```python
from build123d import *

# Parameters (mm, degrees)
ESQUISSE1_W             = 40
ESQUISSE1_H             = 20
BOSS_EXTRU_1_DEPTH      = 2
ESQUISSE2_W             = 40
ESQUISSE2_H             = 2
BOSS_EXTRU_2_DEPTH      = 18
ESQUISSE3_R             = 3
ENL_V_MAT_EXTRU_1_DEPTH = 18
ESQUISSE4_R             = 3
ENL_V_MAT_EXTRU_2_DEPTH = 18
ESQUISSE5_R             = 3
ENL_V_MAT_EXTRU_3_DEPTH = 18
ESQUISSE6_R             = 3
ENL_V_MAT_EXTRU_4_DEPTH = 18
ESQUISSE7_W             = 6
ESQUISSE7_H             = 18
BOSS_EXTRU_3_DEPTH      = 18
ESQUISSE8_R             = 3
ENL_V_MAT_EXTRU_5_DEPTH = 18
CHANFREIN1_SIZE         = 3
CONG_1_R                = 3


with BuildPart() as part:
    # Esquisse1 → Boss.-Extru.1 (new body)
    with BuildSketch(Plane.XY):
        with Locations((-20, 10)):
            Rectangle(ESQUISSE1_W, ESQUISSE1_H)
    extrude(amount=BOSS_EXTRU_1_DEPTH)

    # Esquisse2 → Boss.-Extru.2 (add)
    with BuildSketch(Plane.XY.offset(2)):
        with Locations((-20, 1)):
            Rectangle(ESQUISSE2_W, ESQUISSE2_H)
    extrude(amount=BOSS_EXTRU_2_DEPTH)

    # Esquisse3 → Enlèv. mat.-Extru.1 (cut)
    with BuildSketch(Plane.XY.offset(2)):
        with Locations((-6, 10)):
            Circle(ESQUISSE3_R)
    extrude(amount=-ENL_V_MAT_EXTRU_1_DEPTH, mode=Mode.SUBTRACT)

    # Esquisse4 → Enlèv. mat.-Extru.2 (cut)
    with BuildSketch(Plane.XY.offset(2)):
        with Locations((-25, 10)):
            Circle(ESQUISSE4_R)
    extrude(amount=-ENL_V_MAT_EXTRU_2_DEPTH, mode=Mode.SUBTRACT)

    # Esquisse5 → Enlèv. mat.-Extru.3 (cut)
    with BuildSketch(Plane(origin=(0, 2, 0), x_dir=(1, 0, 0), z_dir=(0, 1, 0))):
        with Locations(Location((-6, -10, 0), (0, 0, 180))):  # turned: the seam where the file's is
            Circle(ESQUISSE5_R)
    extrude(amount=-ENL_V_MAT_EXTRU_3_DEPTH, mode=Mode.SUBTRACT)

    # Esquisse6 → Enlèv. mat.-Extru.4 (cut)
    with BuildSketch(Plane(origin=(0, 2, 0), x_dir=(1, 0, 0), z_dir=(0, 1, 0))):
        with Locations(Location((-25, -10, 0), (0, 0, 180))):  # turned: the seam where the file's is
            Circle(ESQUISSE6_R)
    extrude(amount=-ENL_V_MAT_EXTRU_4_DEPTH, mode=Mode.SUBTRACT)

    # Esquisse7 → Boss.-Extru.3 (add)
    with BuildSketch(Plane(origin=(0, 2, 0), x_dir=(1, 0, 0), z_dir=(0, 1, 0))):
        with Locations((-37, -11)):
            Rectangle(ESQUISSE7_W, ESQUISSE7_H)
    extrude(amount=BOSS_EXTRU_3_DEPTH)

    # Esquisse8 → Enlèv. mat.-Extru.5 (cut)
    with BuildSketch(Plane.ZY.offset(40)):
        with Locations((14, 14)):
            Circle(ESQUISSE8_R)
    extrude(amount=-ENL_V_MAT_EXTRU_5_DEPTH, mode=Mode.SUBTRACT)

    # Chanfrein1
    chanfrein1_edges = [part.edges().sort_by_distance(p)[0] for p in [
        (-37, 20, 20),
    ]]
    chamfer(chanfrein1_edges, length=CHANFREIN1_SIZE)

    # Congé1
    cong_1_edges = [part.edges().sort_by_distance(p)[0] for p in [
        (-34, 11, 2),
    ]]
    fillet(cong_1_edges, radius=CONG_1_R)


solid = part.part
```
Geometry: final body of the model. Coordinates: model frame, mm. A direction names the side the tool comes from. Coordinates: 2 decimals unless noted, no trailing zeros. Order: outer loops, then holes, each group sorted by start corner. A loop starts at its lowest first (then second) coordinate and runs counter-clockwise, first axis right, second up. Notation, with made-up numbers: (-23, -31.75) - (24, -31.75) arc R15 ccw to (24, -21.75) - close; hole circle Ø4 at (78, -15). An arc over 180 degrees is marked (long way). Return JSON: item names as keys, results as strings. Group by question number.
1. Pin query (flat end, axial travel): pin 1 (7 mm diameter, centred on x = -6, z = 10, fed in from +Y); pin 2 (9.5 mm diameter, centred on y = 14, z = 14, fed in from +X); pin 3 (5.5 mm diameter, centred on x = -12, y = 8, fed in from +Z). Return the tip coordinate at first contact, or that it passes through.
2. Cut plane A-A (y = 14). Output: boundary loops of the cut face in (x, z).
3. Pull-direction query (Y, two-part tool) for faces 1 (the face through (-20, 10, 0)), 2 (the face through (-3.14, 10.9, 1.01)), 3 (the face through (-37, 12.2, 11.6)), 4 (the face through (-30.5, 20, 1.5)); classes: pulls with the +Y half, pulls with the -Y half, needs draft (parallel to the pull), parting line crosses it, or undercut.
4. Cut plane D-D (x = -6). Output: boundary loops of the cut face in (y, z).
5. Material intervals for line 1 along Y through (x, z) = (-6, 0.9); line 2 along X through (y, z) = (9, 16), sorted ascending. Write a range as [from, to].
6. Set-up query: faces 5 (the face through (-22, 1, 10)), 6 (the face through (-34, 11, 13)). Return all of +Z, -Z, +X, -X, +Y, -Y with unobstructed straight access to the full face (end or side cutting, diameter ignored); none if empty.
7. Cut plane C-C (y = 10). Output: boundary loops of the cut face in (x, z).
8. Cut plane B-B (z = 14). Output: boundary loops of the cut face in (x, y), plus the area to 3 significant figures.
Resolved:
{
 "1": {"pin 1": "stops at y = 2", "pin 2": "stops at x = -34", "pin 3": "stops at z = 2"},
 "2": {"outline": "(-40, 0) - (0, 0) - (0, 2) - (-31, 2) arc R3 cw to (-34, 5) - (-34, 11) - (-40, 11) - close; (-40, 17) - (-34, 17) - (-34, 20) - (-40, 20) - close"},
 "3": {"face 1": "needs draft", "face 2": "undercut", "face 3": "undercut", "face 4": "pulls with the +Y half"},
 "4": {"outline": "(0, 0) - (7, 0) - (7, 2) - (2, 2) - (2, 7) - (0, 7) - close; (0, 13) - (2, 13) - (2, 20) - (0, 20) - close; (13, 0) - (20, 0) - (20, 2) - (13, 2) - close"},
 "5": {"line 1": "y = [0, 7], [13, 20]", "line 2": "x = [-40, -34]"},
 "6": {"face 5": "+Y, -Y", "face 6": "+Z, +X, +Y"},
 "7": {"outline": "(-40, 0) - (-28, 0) - (-28, 2) - (-31, 2) arc R3 cw to (-34, 5) - (-34, 20) - (-40, 20) - close; (-22, 0) - (-9, 0) - (-9, 2) - (-22, 2) - close; (-3, 0) - (0, 0) - (0, 2) - (-3, 2) - close"},
 "8": {"outline": "(-40, 0) - (0, 0) - (0, 2) - (-34, 2) - (-34, 11) - (-40, 11) - close; (-40, 17) - (-34, 17) - (-34, 20) - (-40, 20) - close", "area": "152 mm²"}
}
